Design review of the part built by this model. Coordinates are the model's own, in mm. Face numbers are marked on the shaded views. A direction names the side the tool comes from. Give positions to 0.01 mm unless a question says otherwise; leave off trailing zeros. Order: outer loops, then holes, each group sorted by start corner. A loop starts at its lowest first (then second) coordinate and runs counter-clockwise, first axis right, second up. Notation, with made-up numbers: M 20,1 L 42,1 A10 cw 42,9 Z; hole C 4,3 d7. An arc over 180 degrees is marked long. Answer as a JSON object with one key per item and string values.
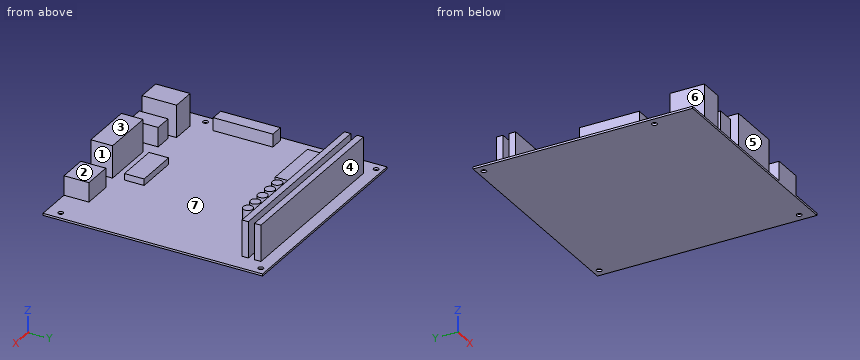
from build123d import *

# Parameters (mm, degrees)
F0_W     = 170
F0_H     = 170
F0_R     = 2
F1_DEPTH = 1.6
F2_W     = 140
F2_H     = 5
F3_DEPTH = 28
F2_W_2   = 18.561
F2_H_2   = 26.719725
F2_W_3   = 41.82321
F2_H_3   = 16.820741
F4_DEPTH = 25
F2_W_4   = 13.611103
F2_H_4   = 22.265183
F2_W_5   = 23.015141
F2_H_5   = 19.295486
F5_DEPTH = 15
F2_R     = 3.769423
F6_DEPTH = 10
F2_W_6   = 33.560348
F2_H_6   = 15.207031
F2_W_7   = 44.047956
F2_H_7   = 22.023975
F7_DEPTH = 5
F2_W_8   = 10.225419
F2_H_8   = 46.145479
F8_DEPTH = 10


with BuildPart() as f1:
    # F0 (on Top) → F1 (new body)
    with BuildSketch(Plane.XY):
        with Locations((44.239621, 37.176466)):
            Rectangle(F0_W, F0_H)
        with Locations((-34.590379, -14.803534)):
            Circle(F0_R, mode=Mode.SUBTRACT)
        with Locations((122.889621, -37.663534)):
            Circle(F0_R, mode=Mode.SUBTRACT)
        with Locations((-34.590379, 117.276466)):
            Circle(F0_R, mode=Mode.SUBTRACT)
        with Locations((122.889621, 117.276466)):
            Circle(F0_R, mode=Mode.SUBTRACT)
    extrude(amount=F1_DEPTH)

    # F2 (on face) → F3 (join)
    with BuildSketch(Plane.XY.offset(1.6)):
        with Locations((44.780245, 100.497786)):
            Rectangle(F2_W, F2_H)
        with Locations((44.780245, 110.224786)):
            Rectangle(F2_W, F2_H)
    extrude(amount=F3_DEPTH)

    # F2 (on face) → F4 (join)
    with BuildSketch(Plane.XY.offset(1.6)):
        with Locations((-15.401558, -34.463671)):
            Rectangle(F2_W_2, F2_H_2)
        with Locations((43.002247, -39.413163)):
            Rectangle(F2_W_3, F2_H_3)
    extrude(amount=F4_DEPTH)

    # F2 (on face) → F5 (join)
    with BuildSketch(Plane.XY.offset(1.6)):
        with Locations((4.396209, -36.690942)):
            Rectangle(F2_W_4, F2_H_4)
        with Locations((89.032523, -38.175791)):
            Rectangle(F2_W_5, F2_H_5)
    extrude(amount=F5_DEPTH)

    # F2 (on face) → F6 (join)
    with BuildSketch(Plane.XY.offset(1.6)):
        with Locations((30.100717, 77.391095)):
            Circle(F2_R)
        with Locations((40.100717, 77.391095)):
            Circle(F2_R)
        with Locations((50.100717, 77.391095)):
            Circle(F2_R)
        with Locations((60.100717, 77.391095)):
            Circle(F2_R)
        with Locations((70.100717, 77.391095)):
            Circle(F2_R)
    extrude(amount=F6_DEPTH)

    # F2 (on face) → F7 (join)
    with BuildSketch(Plane.XY.offset(1.6)):
        with Locations((45.419478, -15.130484)):
            Rectangle(F2_W_6, F2_H_6)
        with Locations((-5.707614, 78.995801)):
            Rectangle(F2_W_7, F2_H_7)
    extrude(amount=F7_DEPTH)

    # F2 (on face) → F8 (join)
    with BuildSketch(Plane.XY.offset(1.6)):
        with Locations((-31.79554, 18.692056)):
            Rectangle(F2_W_8, F2_H_8)
    extrude(amount=F8_DEPTH)


solid = f1.part
(1) We need section C-C (z = 9). Count the separate pieces of the cut face and the enclosed holes in it, plus the area to 3 significant figures.
Checked values:
{"separate pieces": "12", "enclosed holes": "0", "area": "4,040 mm^2"}
(2) We need section D-D (y = 38). Write out the cut boundary in (x, z), plus the area to 3 significant figures.
Checked values:
{"outline": "M -40.76,0 L 129.24,0 L 129.24,1.6 L -26.68,1.6 L -26.68,11.6 L -36.91,11.6 L -36.91,1.6 L -40.76,1.6 Z", "area": "374 mm^2"}
(3) Tool access review of the marked faces 1, 2 and 3: name each direction out of +Z, -Z, +X, -X, +Y, -Y from which nothing blocks a thin tool from reaching the whole face with its end or side.
Checked values:
{"face 1": "+Z, -Y", "face 2": "+Z, +X, -Y", "face 3": "+Z, +X, -X, -Y"}
(4) We need section A-A (z = 19.5). Write out the cut boundary in (x, y), plus the area to 3 significant figures.
Checked values:
{"outline": "M -25.22,98 L 114.78,98 L 114.78,103 L -25.22,103 Z; M -25.22,107.72 L 114.78,107.72 L 114.78,112.72 L -25.22,112.72 Z; M -24.68,-47.82 L -6.12,-47.82 L -6.12,-21.1 L -24.68,-21.1 Z; M 22.09,-47.82 L 63.91,-47.82 L 63.91,-31 L 22.09,-31 Z", "area": "2,600 mm^2"}
(5) To check wall thickness, follow L1, parallel to Y at x = -11, z = 22.5; L2, parallel to Y at x = 25.5, z = 5; L3, parallel to Y at x = -11.5, z = 6.25. State the ranges of each line that lie inside material, in increasing order. Write a range as from..to.
Checked values:
{"L1": "y = -47.82..-21.1, 98..103, 107.72..112.72", "L2": "y = -47.82..-31, 98..103, 107.72..112.72", "L3": "y = -47.82..-21.1, 67.98..90.01, 98..103, 107.72..112.72"}
(6) We need section B-B (x = 103). Write out the cut boundary in (y, z).
Checked values:
{"outline": "M -47.82,0 L 122.18,0 L 122.18,1.6 L 112.72,1.6 L 112.72,29.6 L 107.72,29.6 L 107.72,1.6 L 103,1.6 L 103,29.6 L 98,29.6 L 98,1.6 L -47.82,1.6 Z"}
(7) Insertion check: pin 1 (13.5 mm diameter, centred on y = -39, z = 17, fed in from +X); pin 2 (1.5 mm diameter, centred on y = 76.5, z = 4, fed in from +X); pin 3 (5.5 mm diameter, centred on y = 111, z = 22.5, fed in from -X). Each pin has a flat end and moves straight along its axis. Give the tip position at first contact, or say it passes through.
Checked values:
{"pin 1": "stops at x = 100.54", "pin 2": "stops at x = 73.87", "pin 3": "stops at x = -25.22"}
(8) Draft analysis for pull direction Y (two halves, no side actions). For the marked faces 4, 5, 6 and 7, state which applies: +Y half, -Y half, draft (parallel to the pull), parting line (faces both ways), or undercut.
Checked values:
{"face 4": "+Y half", "face 5": "-Y half", "face 6": "draft", "face 7": "undercut"}
